Answer from the drawing. Dimensions are ordinates in mm from the lowest x, y and z of the part. A direction names the side the tool comes from. Give positions to 0.01 mm unless a question says otherwise; leave off trailing zeros. Write each loop counter-clockwise with the first axis right and the second up, starting at its lowest first coordinate (ties: lowest second). Pieces come first, ordered by that corner, then holes. Notation, with made-up numbers: (44, 77.5) -> (48, 77.5) arc R14 cw to (48, 85.5) -> close; hole circle Ø9 at (52, 47.25). An arc over 180 degrees is marked (long way). Use a Markdown table: item, result. Add a question column.
Q1. Section C-C, the plane y = 22 is taken. Give the vertices of the cut face in (x, z).
Q2. Each of these flat-tipped pins is pushed along its axis until it touches: pin 1 Ø6 at (y, z) = (39.5, 22) entering from -X; pin 2 Ø10 at (x, y) = (45.5, 10.5) entering from -Z (1 decimal); pin 3 Ø6 at (x, z) = (45.5, 14) entering from +Y; pin 4 Ø3 at (y, z) = (13.25, 37.16) entering from +X. Where does it stop, or does it pass through?
Q3. Section D-D, the plane y = 39.5 is taken. Give the vertices of the cut face in (x, z).
Q4. Section B-B, the plane y = 13.25 is taken. Give the vertices of the cut face in (x, z) (1 decimal).
Q5. For the marked faces 1, 2 and 3, determine the directions among +Z, -Z, +X, -X, +Y, -Y from which every point of the face is accessible in a straight line to the end or side of a thin tool.
Q6. Section A-A, the plane z = 22 is taken. Give the vertices of the cut face in (x, y), plus the area to 3 significant figures.
Q7. Consider line 1 (Y direction, x = 14.35, z = 22); line 2 (Z direction, x = 14, y = 13) (1 decimal); line 3 (X direction, y = 29.5, z = 27). Determine where each line is inside the solid, lowest interval first.
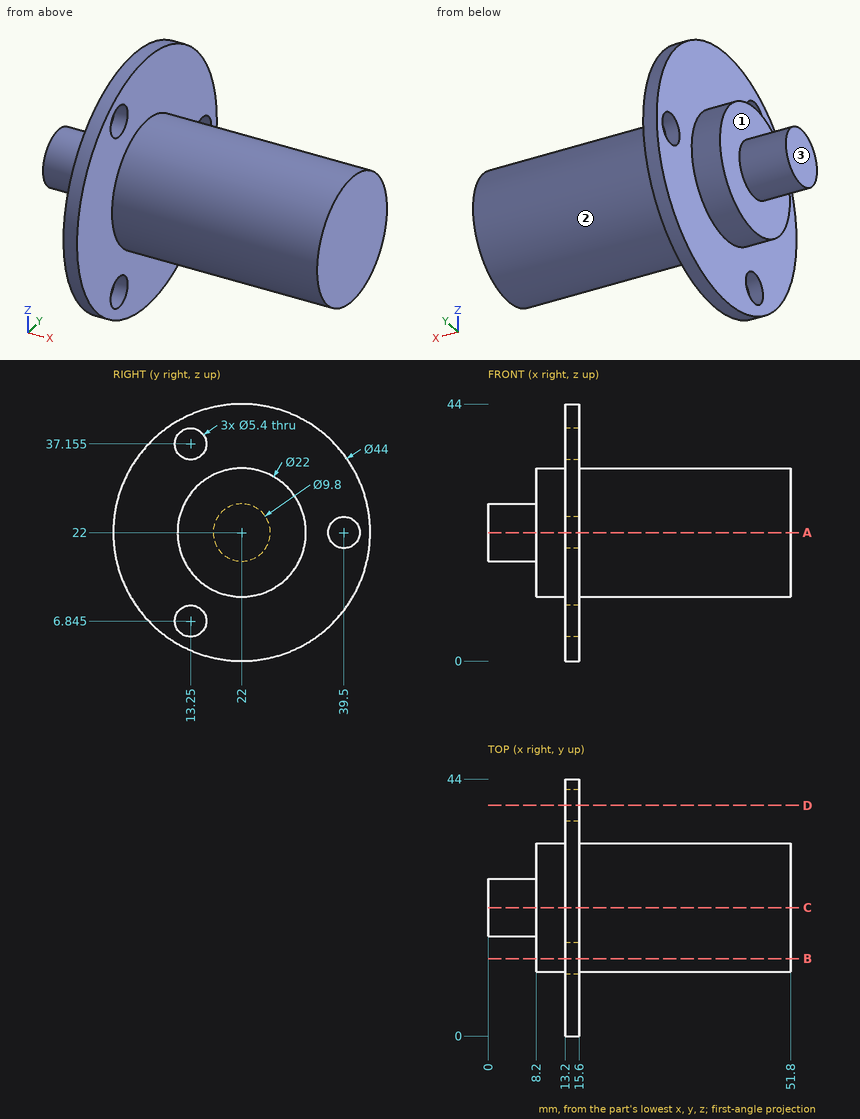
Result set:
| question | item | result |
|---|---|---|
| 1 | outline | (0, 17.1) -> (8.2, 17.1) -> (8.2, 11) -> (13.2, 11) -> (13.2, 0) -> (15.6, 0) -> (15.6, 11) -> (51.8, 11) -> (51.8, 33) -> (15.6, 33) -> (15.6, 44) -> (13.2, 44) -> (13.2, 33) -> (8.2, 33) -> (8.2, 26.9) -> (0, 26.9) -> close |
| 2 | pin 1 | stops at x = 13.2 |
| 2 | pin 2 | stops at z = 13.1 |
| 2 | pin 3 | stops at y = 31.8 |
| 2 | pin 4 | passes through |
| 3 | outline | (13.2, 8.67) -> (15.6, 8.67) -> (15.6, 19.3) -> (13.2, 19.3) -> close; (13.2, 24.7) -> (15.6, 24.7) -> (15.6, 35.33) -> (13.2, 35.33) -> close |
| 4 | outline | (8.2, 15.3) -> (13.2, 15.3) -> (13.2, 9.5) -> (15.6, 9.5) -> (15.6, 15.3) -> (51.8, 15.3) -> (51.8, 28.7) -> (15.6, 28.7) -> (15.6, 34.5) -> (13.2, 34.5) -> (13.2, 28.7) -> (8.2, 28.7) -> close; (13.2, 1.8) -> (15.6, 1.8) -> (15.6, 4.1) -> (13.2, 4.1) -> close; (13.2, 39.9) -> (15.6, 39.9) -> (15.6, 42.2) -> (13.2, 42.2) -> close |
| 5 | face 1 | -X |
| 5 | face 2 | +X |
| 5 | face 3 | +Z, -Z, -X, +Y, -Y |
| 6 | outline | (0, 17.1) -> (8.2, 17.1) -> (8.2, 11) -> (13.2, 11) -> (13.2, 0) -> (15.6, 0) -> (15.6, 11) -> (51.8, 11) -> (51.8, 33) -> (15.6, 33) -> (15.6, 36.8) -> (13.2, 36.8) -> (13.2, 33) -> (8.2, 33) -> (8.2, 26.9) -> (0, 26.9) -> close; (13.2, 42.2) -> (15.6, 42.2) -> (15.6, 44) -> (13.2, 44) -> close |
| 6 | area | 1,080 mm2 |
| 7 | line 1 | y = 0 to 36.8, 42.2 to 44 |
| 7 | line 2 | z = 1.9 to 4.2, 9.5 to 34.5, 39.8 to 42.1 |
| 7 | line 3 | x = 8.2 to 51.8 |
